Source: CAD feature listing. Evaluate the final solid. Frame: model axes, mm. A direction names the side the tool comes from. Give positions to 0.01 mm unless a question says otherwise; leave off trailing zeros. Order: outer loops, then holes, each group sorted by start corner. A loop starts at its lowest first (then second) coordinate and runs counter-clockwise, first axis right, second up. Notation, with made-up numbers: M 28,52.25 L 73,52.25 A20 ccw 73,86.25 Z; hole C -6.75,53.25 d3. An arc over 180 degrees is marked long. Return JSON: item names as keys, results as strings.
from build123d import *

# Parameters (mm, degrees)
BOSS_EXTRUDE2_DEPTH = 2
SKETCH7_R           = 1
BOSS_EXTRUDE3_DEPTH = 2
FILLET1_R           = 2


with BuildPart() as part:
    # Sketch6 → Boss-Extrude2 (new body)
    with BuildSketch(Plane.XY.offset(2)):
        with BuildLine():
            Line((-47.16876351, -59), (-2.443648629, -59))
            ThreePointArc((-2.443648629, -59), (-2.038405947, -58.914209149), (-1.702695493, -58.671556736))
            ThreePointArc((-1.702695493, -58.671556736), (32.301028127, -25.886609728), (70.398776732, 2.035917408))
            ThreePointArc((70.398776732, 2.035917408), (70.813266743, 3.192601161), (69.793484422, 3.877993962))
            Line((69.793484422, 3.877993962), (0.723267865, -0.951866082))
            ThreePointArc((0.723267865, -0.951866082), (0.415830952, -1.023295613), (0.145969905, -1.186986325))
            ThreePointArc((0.145969905, -1.186986325), (-26.215640884, -25.687788129), (-50.262327585, -52.46428288))
            ThreePointArc((-50.262327585, -52.46428288), (-50.784207361, -56.711305279), (-47.16876351, -59))
        make_face()
        with BuildLine():
            Line((-47.16876351, -58), (-2.443648629, -58))
            ThreePointArc((-2.443648629, -58), (31.656951696, -25.121648584), (69.863240895, 2.880429912))
            Line((69.863240895, 2.880429912), (0.793024339, -1.949430132))
            ThreePointArc((0.793024339, -1.949430132), (-25.502517251, -26.388826418), (-49.488936566, -53.09821216))
            ThreePointArc((-49.488936566, -53.09821216), (-49.880346398, -56.28347896), (-47.16876351, -58))
        make_face(mode=Mode.SUBTRACT)
    extrude(amount=BOSS_EXTRUDE2_DEPTH)

    # Sketch7 → Boss-Extrude3 (add)
    with BuildSketch(Plane.XY.offset(4)):
        with BuildLine():
            Line((73.71668331, 5.154772651), (0.326528995, 0.022833132))
            ThreePointArc((0.326528995, 0.022833132), (0.019473004, -0.048441349), (-0.250141607, -0.211755142))
            ThreePointArc((-0.250141607, -0.211755142), (-26.813414366, -24.869459397), (-51.035718603, -51.8303536))
            ThreePointArc((-51.035718603, -51.8303536), (-51.688068324, -57.139131599), (-47.16876351, -60))
            Line((-47.16876351, -60), (-2, -60))
            Line((-2, -60), (-2, -59))
            ThreePointArc((-2, -59), (33.663262979, -24.745525454), (73.786439783, 4.157208601))
            Line((73.786439783, 4.157208601), (73.71668331, 5.154772651))
        make_face()
        with Locations((58.629217017, -0.912455258)):
            Circle(SKETCH7_R, mode=Mode.SUBTRACT)
        with Locations((-47.16876351, -55)):
            Circle(SKETCH7_R, mode=Mode.SUBTRACT)
    extrude(amount=BOSS_EXTRUDE3_DEPTH)

    # Fillet1
    fillet1_edges = [part.edges().sort_by_distance(p)[0] for p in [
        (69.863240895, 2.880429912, 3),
        (0.793024339, -1.949430132, 3),
        (-2.443648629, -58, 3),
    ]]
    fillet(fillet1_edges, radius=FILLET1_R)


solid = part.part
1. Ray query, probe 1 along X at (y, z) = (-8, 3.25); probe 2 along X at (y, z) = (-18.5, 3); probe 3 along Y at (x, z) = (28, 3.35). Return the intervals inside material, ascending.
Evaluation:
{"probe 1": "x = -7.67 to -6.17, 53.71 to 55.44", "probe 2": "x = -18.97 to -17.53, 39.76 to 41.38", "probe 3": "y = -29.57 to -28.24, -0.05 to 0.96"}
2. Set-up query: faces 4 (the face through (28.599, -27.726, 2.986)), 5 (the face through (-50.811, -56.654, 2.986)), 6 (the face through (-25.862, -25.329, 2.986)), 7 (the face through (-51.72, -57.07, 4.99)). Return all of +Z, -Z, +X, -X, +Y, -Y with unobstructed straight access to the full face (end or side cutting, diameter ignored); none if empty.
Evaluation:
{"face 4": "-Z", "face 5": "-Z, -X", "face 6": "-Z, -X, +Y", "face 7": "+Z, -Z, -X"}
3. Section query B-B (x = -17.5). Return loops of the section in (y, z), then the cut area to 3 significant figures.
Evaluation:
{"outline": "M -60,4 L -59,4 L -59,2 L -58,2 L -58,4 L -18.48,4 L -18.48,2 L -17.09,2 L -17.09,4 L -15.71,4 L -15.71,6 L -60,6 Z", "area": "93.4 mm^2"}
4. Section query C-C (y = -42). Return loops of the section in (x, z).
Evaluation:
{"outline": "M -42.71,4 L -41.38,4 L -41.38,2 L -40.05,2 L -40.05,4 L 13.01,4 L 13.01,2 L 14.44,2 L 14.44,6 L -42.71,6 Z"}
5. First-contact query: pin 1 (2.5 mm diameter, centred on x = -47.17, y = -55, fed in from -Z); pin 2 (2 mm diameter, centred on x = 12.5, z = 5, fed in from -Y); pin 3 (1 mm diameter, centred on x = -24.5, z = 3, fed in from -Y). Flat tips, straight axial feed; report the tip coordinate or a pass-through.
Evaluation:
{"pin 1": "stops at z = 4", "pin 2": "stops at y = -44.88", "pin 3": "stops at y = -59"}
6. Section query A-A (z = 2.6). Return loops of the section in (x, y), then the cut area to 3 significant figures.
Evaluation:
{"outline": "M -50.26,-52.46 A4 ccw -47.17,-59 L -2.44,-59 A1 ccw -1.7,-58.67 A351 cw 70.4,2.04 A1 ccw 69.79,3.88 L 0.72,-0.95 A1 ccw 0.15,-1.19 A399 ccw Z; hole M -49.49,-53.1 A3 ccw -47.17,-58 L -3.33,-58 A2 ccw -1.85,-57.35 A352 cw 63.4,-1.32 A2 ccw 62.15,2.34 L 1.45,-1.9 A2 ccw 0.29,-2.38 A398 ccw Z", "area": "301 mm^2"}
7. Draft query along Y for faces 1 (the face through (32.22, 0.25, 2.99)), 2 (the face through (35.742, 1.497, 2.986)), 3 (the face through (1.2, -0.7, 4)). Return one class per face: pulls with the +Y half, pulls with the -Y half, needs draft (parallel to the pull), parting line crosses it, or undercut.
Evaluation:
{"face 1": "undercut", "face 2": "pulls with the +Y half", "face 3": "needs draft"}
8. Section query D-D (x = 25.5). Return loops of the section in (y, z), then the cut area to 3 significant figures.
Evaluation:
{"outline": "M -31.76,2 L -30.43,2 L -30.43,4 L -0.22,4 L -0.22,2 L 0.78,2 L 0.78,4 L 1.78,4 L 1.78,6 L -31.76,6 Z", "area": "71.8 mm^2"}
